Study the drawing (mm; zero at the part's minimum x, y, z) and answer. A direction names the side the tool comes from. Round coordinates to 2 decimals unless told otherwise and drop trailing zeros. Write each loop counter-clockwise with the first axis right and the second up, starting at its lowest first coordinate (ties: lowest second). Pieces come first, ordered by that corner, then holes. Notation, with made-up numbers: (65.25, -1) - (77.25, -1) arc R31 cw to (77.25, 38) - close; hole circle Ø11 at (40.5, 54). An arc over 180 degrees is marked (long way). Return JSON: item names as keys, results as strings. Group by question number.
(1) Which of the six approach directions +Z, -Z, +X, -X, +Y, -Y give full straight-line access (tool end or side, diameter ignored) to the marked faces 4, 5, 6, 7 and 8?
(2) Find the intervals of material crossed by line 1 along X through (y, z) = (22.5, 47); line 2 along Y through (x, z) = (134, 35.5); line 3 along Z through (x, y) = (134.5, 39), in increasing order. Write a range as [from, to].
(3) Section B-B, the plane y = 52.5 is taken. Write down the section's boundary in (x, z), then the cut area to 3 significant figures.
(4) Section D-D, the plane y = 36 is taken. Write down the section's boundary in (x, z).
(5) Determine the mould class of the marked faces 1, 2 and 3 for opening direction X: +X half, -X half, draft (parallel to the pull), parting line (faces both ways), or undercut.
(6) Section C-C, the plane z = 18 is taken. Write down the section's boundary in (x, y), then the cut area to 3 significant figures.
(7) Each of these flat-tipped pins is pushed along its axis until it touches: pin 1 (9 mm diameter, centred on x = 29.5, y = 16.5, fed in from +Z); pin 2 (1 mm diameter, centred on x = 76.5, y = 45.5, fed in from +Z); pin 3 (22 mm diameter, centred on y = 9.5, z = 71, fed in from -X); pin 4 (18 mm diameter, centred on x = 104.5, z = 64, fed in from -Y). Where does it stop, or does it pass through?
(8) Section A-A, the plane x = 67.5 is taken. Write down the section's boundary in (y, z).
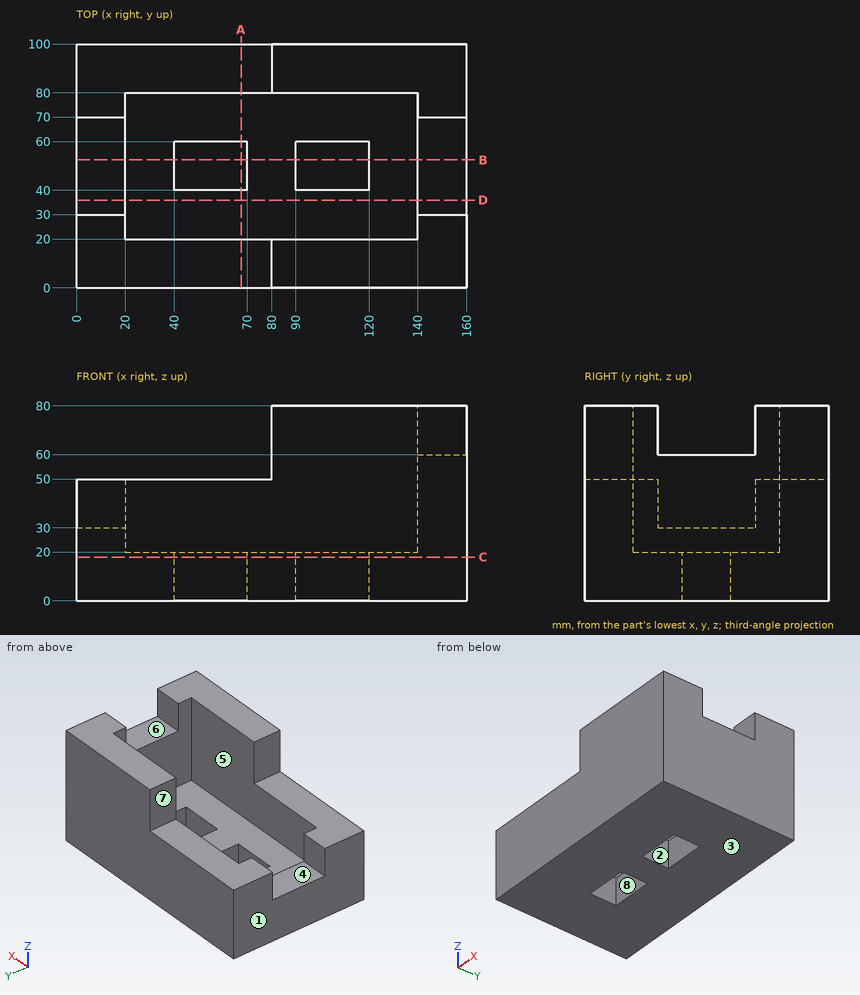
Working result:
{
 "1": {"face 4": "+Z, -X", "face 5": "+Z", "face 6": "+Z, +X, -X", "face 7": "+Z, -X, +Y, -Y", "face 8": "+Z, -Z"},
 "2": {"line 1": "x = [0, 20], [140, 160]", "line 2": "y = [0, 20], [80, 100]", "line 3": "z = [0, 20]"},
 "3": {"outline": "(0, 0) - (40, 0) - (40, 20) - (20, 20) - (20, 30) - (0, 30) - close; (70, 0) - (90, 0) - (90, 20) - (70, 20) - close; (120, 0) - (160, 0) - (160, 60) - (140, 60) - (140, 20) - (120, 20) - close", "area": "3,000 mm^2"},
 "4": {"outline": "(0, 0) - (160, 0) - (160, 60) - (140, 60) - (140, 20) - (20, 20) - (20, 30) - (0, 30) - close"},
 "5": {"face 1": "-X half", "face 2": "undercut", "face 3": "draft"},
 "6": {"outline": "(0, 0) - (160, 0) - (160, 100) - (0, 100) - close; hole (40, 40) - (70, 40) - (70, 60) - (40, 60) - close; hole (90, 40) - (120, 40) - (120, 60) - (90, 60) - close", "area": "14,800 mm^2"},
 "7": {"pin 1": "stops at z = 50", "pin 2": "stops at z = 20", "pin 3": "stops at x = 80", "pin 4": "stops at y = 0"},
 "8": {"outline": "(0, 0) - (40, 0) - (40, 20) - (20, 20) - (20, 50) - (0, 50) - close; (60, 0) - (100, 0) - (100, 50) - (80, 50) - (80, 20) - (60, 20) - close"}
}
